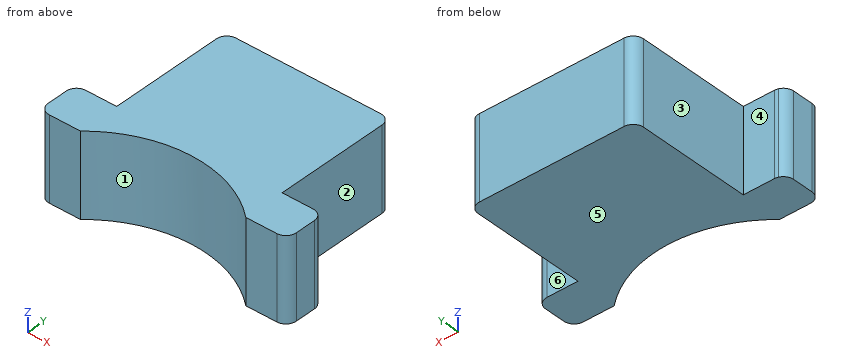
from build123d import *

# Parameters (mm, degrees)
F1_DEPTH = 40


with BuildPart() as f1:
    # F0 (on Top) → F1 (new body)
    with BuildSketch(Plane.XY):
        with BuildLine():
            Line((75, 80), (5, 80))
            ThreePointArc((5, 80), (1.464466, 78.535534), (0, 75))
            Line((0, 75), (0, 20))
            Line((0, 20), (-15, 20))
            ThreePointArc((-15, 20), (-15.914796, 19.915603), (-16.798709, 19.66526))
            ThreePointArc((-16.798709, 19.66526), (-19.122714, 17.828998), (-20, 15))
            Line((-20, 15), (-20, 5))
            ThreePointArc((-20, 5), (-18.535534, 1.464466), (-15, 0))
            Line((-15, 0), (0, 0))
            ThreePointArc((0, 0), (40, 15.263289), (80, 0))
            Line((80, 0), (95, 0))
            ThreePointArc((95, 0), (98.535534, 1.464466), (100, 5))
            Line((100, 5), (100, 15))
            ThreePointArc((100, 15), (98.535534, 18.535534), (95, 20))
            Line((95, 20), (80, 20))
            Line((80, 20), (80, 75))
            ThreePointArc((80, 75), (78.535534, 78.535534), (75, 80))
        make_face()
    extrude(amount=F1_DEPTH)


solid = f1.part
Here's how the part is built. I have some questions about the finished solid (model axes, mm). Face numbers are marked on the shaded views. A direction names the side the tool comes from. Coordinates: 2 decimals unless noted, no trailing zeros. Loops run counter-clockwise (first coordinate to the right, second up) from the corner with the lowest first, then second, coordinate; pieces in that order, holes last.
1. Imagine slicing it at B-B, the plane y = 36.5. Please give me the cut outline in (x, z).
2. For P1, Ø16.5, axis at x = -10, z = 12.5, coming from the +Y side; P2, Ø8, axis at y = 42, z = 6, coming from the +X side; P3, Ø1, axis at x = 81.5, y = 50, coming from the +Z side; P4, Ø2, axis at y = 26.5, z = 14.5, coming from the -X side, each with a flat end and sliding along its axis, tell me the tip position at first contact or that it passes through.
3. If we mould it in two halves opening along X, with no side actions, what happens to the marked faces 1, 2 and 3? For each: pulls with the +X half, pulls with the -X half, needs draft (parallel to the pull), parting line crosses it, or undercut.
4. For the marked faces 4, 5 and 6, which set-ups out of +Z, -Z, +X, -X, +Y, -Y let a thin tool reach every point of the face, with its end or its side?
5. I need wall thicknesses on L1, parallel to X at y = 25, z = 15.5; L2, parallel to X at y = 11, z = 28.5; L3, parallel to X at y = 10.5, z = 13. Which ranges of each line are inside material? Lowest first, please.
6. Imagine slicing it at A-A, the plane z = 31. Please give me the cut outline in (x, y).
7. Imagine slicing it at C-C, the plane x = 14. Please give me the cut outline in (y, z).
Taken from the geometry:
1. outline: (0, 0) - (80, 0) - (80, 40) - (0, 40) - close
2. P1: stops at y = 20
2. P2: stops at x = 80
2. P3: passes through
2. P4: stops at x = 0
3. face 1: undercut
3. face 2: pulls with the +X half
3. face 3: pulls with the -X half
4. face 4: +Z, -Z, -X, +Y
4. face 5: -Z, +X, -X, +Y, -Y
4. face 6: +Z, -Z, +X, +Y
5. L1: x = 0 to 80
5. L2: x = -20 to 17.78, 62.22 to 100
5. L3: x = -20 to 16.56, 63.44 to 100
6. outline: (-20, 5) arc R5 ccw to (-15, 0) - (0, 0) arc R60.04 cw to (80, 0) - (95, 0) arc R5 ccw to (100, 5) - (100, 15) arc R5 ccw to (95, 20) - (80, 20) - (80, 75) arc R5 ccw to (75, 80) - (5, 80) arc R5 ccw to (0, 75) - (0, 20) - (-15, 20) arc R5 ccw to (-16.8, 19.67) arc R5 ccw to (-20, 15) - close
7. outline: (9.34, 0) - (80, 0) - (80, 40) - (9.34, 40) - close
